Job drawing, mm, ordinate dimensions from the low corner. One solid piece. Round coordinates to 2 decimals unless told otherwise and drop trailing zeros. Order: outer loops, then holes, each group sorted by start corner. A loop starts at its lowest first (then second) coordinate and runs counter-clockwise, first axis right, second up. Notation, with made-up numbers: (-19, -25) -> (30, -25) arc R10 ccw to (30, -10) -> close; hole circle Ø2 at (4, 34). An arc over 180 degrees is marked (long way). Write item = value, one per line.
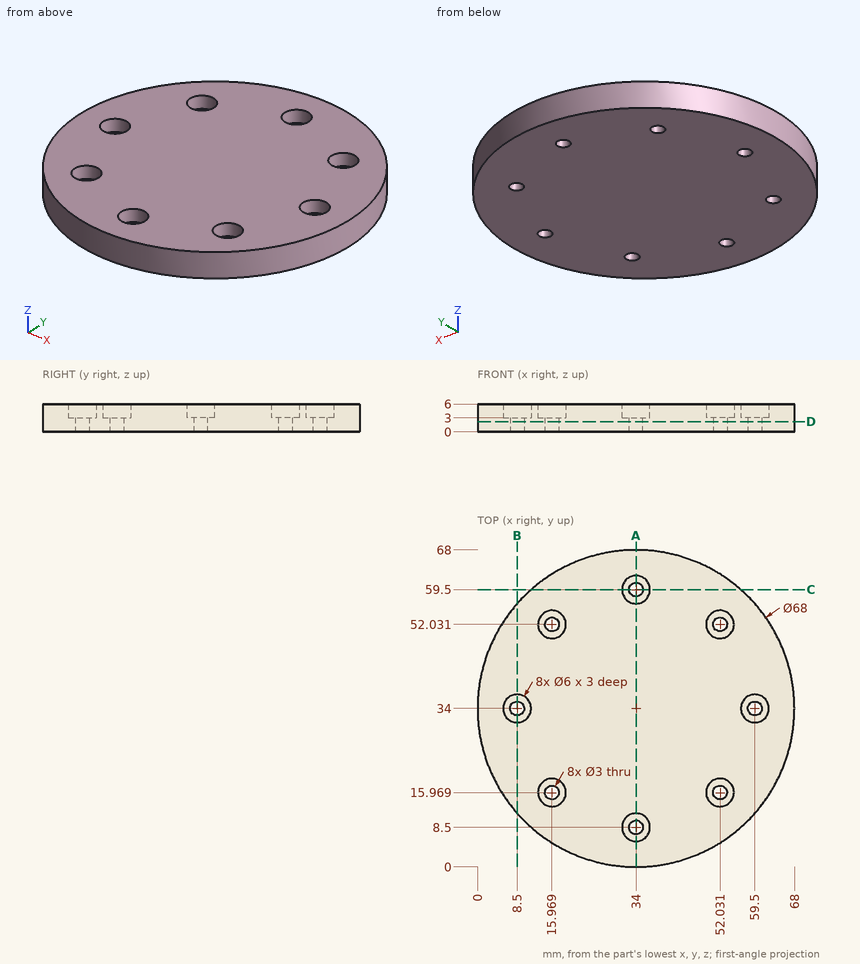
Q1. Probe probe 1 along Y at (x, z) = (16, 5.3) (1 decimal); probe 2 along X at (y, z) = (53.5, 4.95) (1 decimal); probe 3 along Y at (x, z) = (59.5, 2.25). List the from-to ranges inside material, lowest first.
Check values:
probe_1 = 5.2 to 13, 19 to 49, 55 to 62.8
probe_2 = 6.1 to 13.4, 18.6 to 49.4, 54.6 to 61.9
probe_3 = 11.51 to 32.5, 35.5 to 56.49
Q2. Flat gauge pins, fed straight in: pin 1 (1.8 mm diameter, centred on x = 52.03, y = 15.97, fed in from +Z); pin 2 (1.5 mm diameter, centred on y = 26, z = 5.5, fed in from +X); pin 3 (3 mm diameter, centred on x = 59, y = 33.5, fed in from +Z); pin 4 (1 mm diameter, centred on x = 31.5, z = 3, fed in from +Y). Where does each tip first touch, or does it go through?
Check values:
pin_1 = through
pin_2 = 67.22
pin_3 = 3
pin_4 = 67.94
Q3. Cut at D-D, the plane z = 2.2. Give the number of separate pieces and of enclosed holes in the cut face, and give its area (4 significant figures).
Check values:
separate_pieces = 1
enclosed_holes = 8
area = 3,575 mm²
Q4. Cut at A-A, the plane x = 34. List the corners of the cut face in (y, z), and give its area (3 significant figures).
Check values:
outline = (0, 0) -> (7, 0) -> (7, 3) -> (5.5, 3) -> (5.5, 6) -> (0, 6) -> close; (10, 0) -> (58, 0) -> (58, 3) -> (56.5, 3) -> (56.5, 6) -> (11.5, 6) -> (11.5, 3) -> (10, 3) -> close; (61, 0) -> (68, 0) -> (68, 6) -> (62.5, 6) -> (62.5, 3) -> (61, 3) -> close
area = 354 mm²
Q5. Cut at B-B, the plane x = 8.5. List the corners of the cut face in (y, z).
Check values:
outline = (11.51, 0) -> (32.5, 0) -> (32.5, 3) -> (31, 3) -> (31, 6) -> (11.51, 6) -> close; (35.5, 0) -> (56.49, 0) -> (56.49, 6) -> (37, 6) -> (37, 3) -> (35.5, 3) -> close
